from build123d import *

# Parameters (mm, degrees)
SKETCH_1_W          = 50.5
SKETCH_1_H          = 106
EXTRUDE_1_DEPTH     = 10
SKETCH_4_W          = 44.5
SKETCH_4_H          = 100
EXTRUDE_7_DEPTH     = 7
SKETCH_4_4_W        = 44.5
SKETCH_4_4_H        = 100
CUT_EXTRUDE_1_DEPTH = 7.5
SKETCH_6_W          = 13
SKETCH_6_H          = 5
CUT_EXTRUDE_2_DEPTH = 3
SKETCH_7_W          = 13.6
SKETCH_7_H          = 6
SKETCH_7_W_2        = 12
CUT_EXTRUDE_3_DEPTH = 3


with BuildPart() as part:
    # 草图1 → 凸台-拉伸1 (new body)
    with BuildSketch(Plane(origin=(0, 0, 0), x_dir=(1, 0, 0), z_dir=(0, 1, 0))):
        with Locations((4.235483871, -32.8)):
            Rectangle(SKETCH_1_W, SKETCH_1_H)
    extrude(amount=EXTRUDE_1_DEPTH)

    # 草图4 → 凸台-拉伸7 (add)
    with BuildSketch(Plane(origin=(0, 10, 0), x_dir=(1, 0, 0), z_dir=(0, 1, 0))):
        with Locations((4.235483871, -32.8)):
            Rectangle(SKETCH_4_W, SKETCH_4_H)
    extrude(amount=-EXTRUDE_7_DEPTH)

    # 草图4<4> → 切除-拉伸1 (cut)
    with BuildSketch(Plane(origin=(0, 10, 0), x_dir=(1, 0, 0), z_dir=(0, 1, 0))):
        with Locations((4.235483871, -32.8)):
            Rectangle(SKETCH_4_4_W, SKETCH_4_4_H)
    extrude(amount=-CUT_EXTRUDE_1_DEPTH, mode=Mode.SUBTRACT)

    # 草图6 → 切除-拉伸2 (cut)
    with BuildSketch(Plane.ZY.offset(21.014516129)):
        with Locations((-4.7, 5.5)):
            Rectangle(SKETCH_6_W, SKETCH_6_H)
        with Locations((23.3, 5.5)):
            Rectangle(SKETCH_6_W, SKETCH_6_H)
    extrude(amount=-CUT_EXTRUDE_2_DEPTH, mode=Mode.SUBTRACT)

    # 草图7 → 切除-拉伸3 (cut)
    with BuildSketch(Plane(origin=(29.485483871, 0, 0), x_dir=(0, 0, -1), z_dir=(1, 0, 0))):
        with Locations((3.1, 6)):
            Rectangle(SKETCH_7_W, SKETCH_7_H)
        with Locations((-22.5, 6)):
            Rectangle(SKETCH_7_W, SKETCH_7_H)
        with Locations((-48.1, 6)):
            Rectangle(SKETCH_7_W, SKETCH_7_H)
        with Locations((-72.9, 6)):
            Rectangle(SKETCH_7_W_2, SKETCH_7_H)
    extrude(amount=-CUT_EXTRUDE_3_DEPTH, mode=Mode.SUBTRACT)


solid = part.part
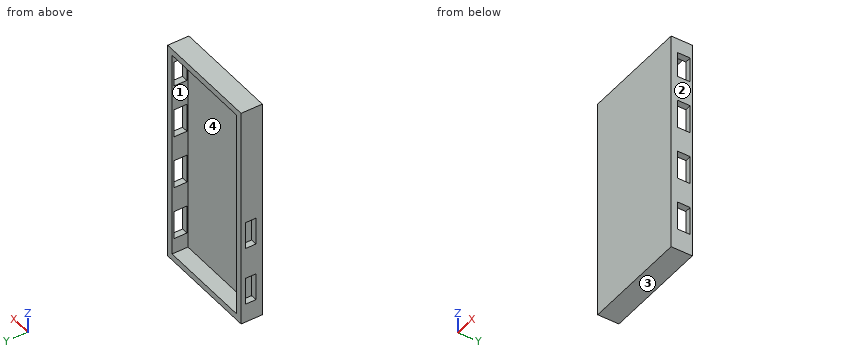
Work out the finished part from the listing and answer in its coordinate system (mm). Face numbers are marked on the shaded views. Coordinates: 2 decimals unless noted, no trailing zeros. Write each loop counter-clockwise with the first axis right and the second up, starting at its lowest first coordinate (ties: lowest second). Pieces come first, ordered by that corner, then holes. Notation, with made-up numbers: M 39.5,66.5 L 60.5,66.5 A26 ccw 60.5,97.5 Z; hole C 4,11.5 d3. An arc over 180 degrees is marked long. Use one line per item in the form item = value. Start each with the question number.
1. Straight lines are drawn through the part: probe 1 along Z at (x, y) = (24, 9); probe 2 along X at (y, z) = (3, 4.5); probe 3 along X at (y, z) = (8.75, -7). For each, find the intervals that lie inside material, in ascending order. Write a range as from..to.
2. This flat-tipped pin is pushed along its axis until it touches: P1, Ø10, axis at x = 12.5, z = 58.5, coming from the +Y side. Where does it stop, or does it pass through?
3. The mould has two halves that part along Z. Classify the marked faces 1, 2, 3 and 4: released by +Z, released by -Z, zero draft, split by the parting line, or undercut.
4. The part is cut by section A-A (y = 4.75). Give the number of separate pieces and of enclosed holes in the cut face, plus the area to 3 significant figures.
5. The part is cut by section B-B (z = 52). Give the vertices of the cut face in (x, y), plus the area to 3 significant figures.
6. The part is cut by section C-C (x = -9). Give the vertices of the cut face in (y, z), plus the area to 3 significant figures.
Evaluation:
q1.probe_1 = -20.2..-17.2, 82.8..85.8
q1.probe_2 = -21.01..-18.01, 26.49..29.49
q1.probe_3 = -21.01..-18.01
q2.P1 = 2.5
q3.face_1 = undercut
q3.face_2 = zero draft
q3.face_3 = released by -Z
q3.face_4 = undercut
q4.separate_pieces = 6
q4.enclosed_holes = 0
q4.area = 667 mm^2
q5.outline = M -21.01,0 L 29.49,0 L 29.49,3 L 26.49,3 L 26.49,2.5 L -18.01,2.5 L -18.01,10 L -21.01,10 Z; M 26.49,9 L 29.49,9 L 29.49,10 L 26.49,10 Z
q5.area = 153 mm^2
q6.outline = M 0,-20.2 L 10,-20.2 L 10,-17.2 L 2.5,-17.2 L 2.5,82.8 L 10,82.8 L 10,85.8 L 0,85.8 Z
q6.area = 310 mm^2
